For this review, use the dimensioned drawing (mm, ordinates from the lowest corner) and the shaded views. Give positions to 0.01 mm unless a question says otherwise; leave off trailing zeros. Loops run counter-clockwise (first coordinate to the right, second up) from the corner with the lowest first, then second, coordinate; pieces in that order, holes last. Notation, with made-up numbers: (-4.75, -12.5) -> (31.25, -12.5) arc R14 ccw to (31.25, -0.5) -> close; hole circle Ø8 at (19.5, 66). An arc over 180 degrees is marked (long way). Write each question's results on one line, items separated by ' | '. Start each with the question number.
Q1. Wall thickness on L1, parallel to Y at x = 6, z = 2.9; L2, parallel to X at y = 54.5, z = 0.6: over which ranges is each line inside the solid? List them lowest first. Write a range as [from, to].
Q2. Insertion check: pin 1 Ø3 at (x, y) = (71, 3.592) entering from +Z; pin 2 Ø1.5 at (x, y) = (49, 32) entering from -Z. Each pin has a flat end and moves straight along its axis. Give the tip position at first contact, or say it passes through.
Q3. We need section A-A (x = 71). Write out the cut boundary in (y, z), plus the area to 3 significant figures.
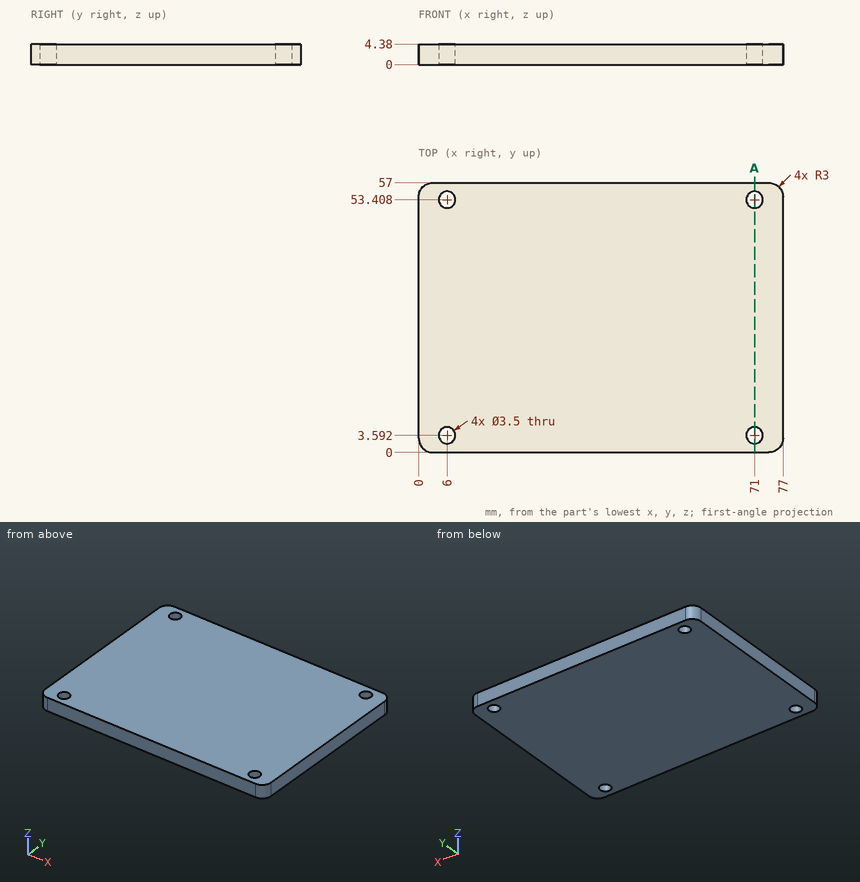
Output:
1) L1: [0, 1.84], [5.34, 51.66], [55.16, 57] | L2: [0.04, 4.63], [7.37, 69.63], [72.37, 76.96]
2) pin 1: through | pin 2: z = 0
3) outline: (0, 0) -> (1.84, 0) -> (1.84, 4.38) -> (0, 4.38) -> close; (5.34, 0) -> (51.66, 0) -> (51.66, 4.38) -> (5.34, 4.38) -> close; (55.16, 0) -> (57, 0) -> (57, 4.38) -> (55.16, 4.38) -> close | area: 219 mm2
